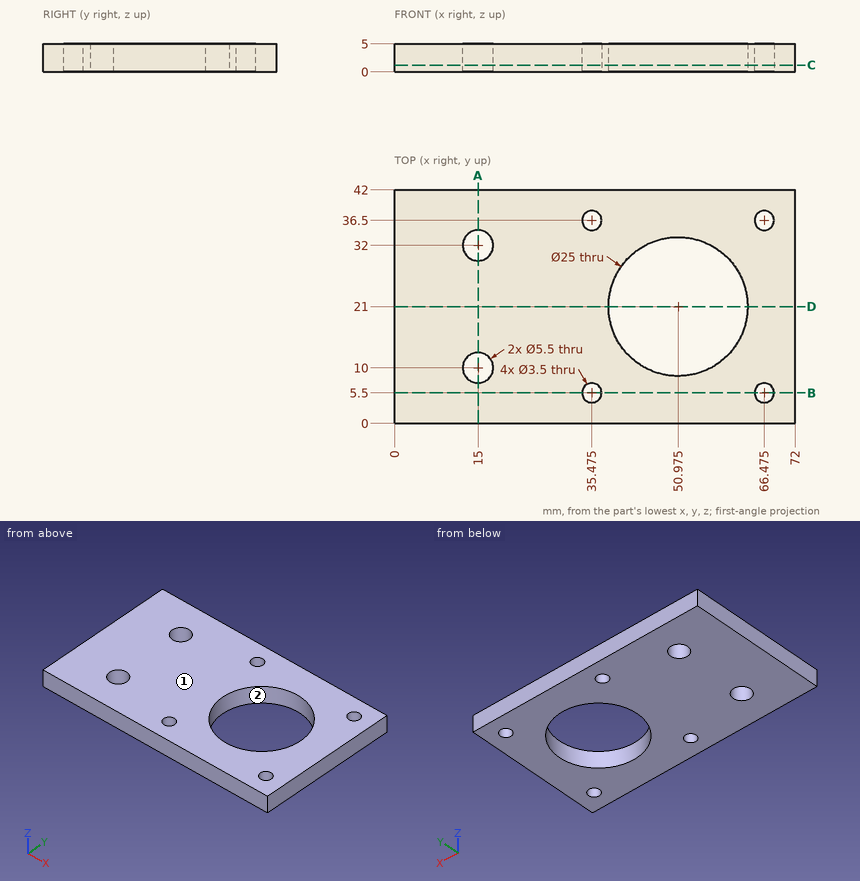
Check sheet for the drawn part. Datum: minimum x, y, z corner. Units: mm. Coordinates: 2 decimals unless noted, no trailing zeros. Write each loop counter-clockwise with the first axis right and the second up, starting at its lowest first coordinate (ties: lowest second). Pieces come first, ordered by that corner, then holes. Notation, with made-up numbers: M 34,-9.5 L 69,-9.5 A17 ccw 69,0.5 Z; hole C 4.25,-23.5 d5. An arc over 180 degrees is marked long. Use a Markdown table: item, result.
Q1. Sectioned sample at A-A, the plane x = 15. Record the boundary of the cut face in (y, z), plus the area to 3 significant figures.
Reply:
| item | result |
|---|---|
| outline | M 0,0 L 7.25,0 L 7.25,5 L 0,5 Z; M 12.75,0 L 29.25,0 L 29.25,5 L 12.75,5 Z; M 34.75,0 L 42,0 L 42,5 L 34.75,5 Z |
| area | 155 mm² |
Q2. Sectioned sample at B-B, the plane y = 5.5. Record the boundary of the cut face in (x, z) (3 decimals), plus the area to 3 significant figures.
Reply:
| item | result |
|---|---|
| outline | M 0,0 L 33.725,0 L 33.725,5 L 0,5 Z; M 37.225,0 L 64.725,0 L 64.725,5 L 37.225,5 Z; M 68.225,0 L 72,0 L 72,5 L 68.225,5 Z |
| area | 325 mm² |
Q3. Sectioned sample at D-D, the plane y = 21. Record the boundary of the cut face in (x, z) (3 decimals).
Reply:
| item | result |
|---|---|
| outline | M 0,0 L 38.475,0 L 38.475,5 L 0,5 Z; M 63.475,0 L 72,0 L 72,5 L 63.475,5 Z |
Q4. Sectioned sample at C-C, the plane z = 1.2. Record the boundary of the cut face in (x, y) (3 decimals).
Reply:
| item | result |
|---|---|
| outline | M 0,0 L 72,0 L 72,42 L 0,42 Z; hole C 15,10 d5.5; hole C 15,32 d5.5; hole C 35.475,5.5 d3.5; hole C 35.475,36.5 d3.5; hole C 50.975,21 d25; hole C 66.475,5.5 d3.5; hole C 66.475,36.5 d3.5 |
Q5. Draft check along X on the marked faces 1 and 2. Enter one of: +X half, -X half, draft (parallel to the pull), parting line (faces both ways), or undercut.
Reply:
| item | result |
|---|---|
| face 1 | draft |
| face 2 | undercut |
Q6. Thickness scan on line 1 (Y direction, x = 15, z = 1.65); line 2 (Y direction, x = 36, z = 2.1); line 3 (X direction, y = 6.5, z = 0.95). Record the ranges inside material, lowest first.
Reply:
| item | result |
|---|---|
| line 1 | y = 0 to 7.25, 12.75 to 29.25, 34.75 to 42 |
| line 2 | y = 0 to 3.83, 7.17 to 34.83, 38.17 to 42 |
| line 3 | x = 0 to 34.04, 36.91 to 65.04, 67.91 to 72 |
